Geometry: final body of the model. Coordinates: model frame, mm. Give positions to 0.01 mm unless a question says otherwise; leave off trailing zeros. Loops run counter-clockwise (first coordinate to the right, second up) from the corner with the lowest first, then second, coordinate; pieces in that order, holes last. Notation, with made-up numbers: (66.5, 71.25) -> (112.5, 71.25) arc R24 ccw to (112.5, 86.25) -> close; hole circle Ø7 at (70.5, -32). An arc over 180 degrees is marked (long way). One line per question, with ' | ' between items. Start each with the question number.
Item 1: Pin query (flat end, axial travel): P1, Ø0.9, axis at x = 2, z = -17, coming from the +Y side; P2, Ø0.9, axis at x = 1, y = 61, coming from the -Z side. Return the tip coordinate at first contact, or that it passes through.
Item 2: Section A-A on z = -3. Give the number of separate pieces and of enclosed holes in the cut face, then the cut area to 4 significant figures.
Item 3: Material intervals for line 1 along Z through (x, y) = (1.45, -81); line 2 along Z through (x, y) = (2.85, -53), sorted ascending. Write a range as [from, to].
Item 4: Section C-C on y = -57.5. Return loops of the section in (x, z).
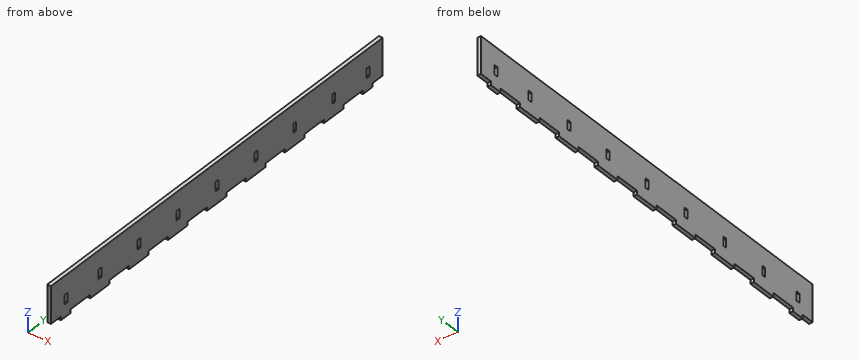
from build123d import *

# Parameters (mm, degrees)
F0_W      = 280
F0_H      = 30
F1_DEPTH  = 3
F2_W      = 20
F2_H      = 3
F3_DEPTH  = 3
F4_W      = 3
F4_H      = 7.5
F5_DEPTH  = 25
F6_W      = 30.25
F6_H      = 30
F7_DEPTH  = 3
F8_W      = 10
F8_H      = 3
F9_DEPTH  = 3
F10_W     = 3
F10_H     = 7.5
F11_DEPTH = 25


with BuildPart() as f1:
    # F0 (on Right) → F1 (new body)
    with BuildSketch(Plane.YZ):
        Rectangle(F0_W, F0_H)
    extrude(amount=F1_DEPTH)

    # F2 (on face) → F3 (join, through all)
    with BuildSketch(Plane.YZ.offset(3)):
        with Locations((120, -16.5)):
            Rectangle(F2_W, F2_H)
        with Locations((80, -16.5)):
            Rectangle(F2_W, F2_H)
        with Locations((40, -16.5)):
            Rectangle(F2_W, F2_H)
        with Locations((0, -16.5)):
            Rectangle(F2_W, F2_H)
        with Locations((-40, -16.5)):
            Rectangle(F2_W, F2_H)
        with Locations((-80, -16.5)):
            Rectangle(F2_W, F2_H)
        with Locations((-120, -16.5)):
            Rectangle(F2_W, F2_H)
    extrude(amount=-F3_DEPTH)

    # F4 (on face) → F5 (cut)
    with BuildSketch(Plane.YZ.offset(3)):
        with Locations((120, -3.75)):
            Rectangle(F4_W, F4_H)
        with Locations((80, -3.75)):
            Rectangle(F4_W, F4_H)
        with Locations((40, -3.75)):
            Rectangle(F4_W, F4_H)
        with Locations((0, -3.75)):
            Rectangle(F4_W, F4_H)
        with Locations((-40, -3.75)):
            Rectangle(F4_W, F4_H)
        with Locations((-80, -3.75)):
            Rectangle(F4_W, F4_H)
        with Locations((-120, -3.75)):
            Rectangle(F4_W, F4_H)
    extrude(amount=-F5_DEPTH, mode=Mode.SUBTRACT)

    # F6 (on face) → F7 (join)
    with BuildSketch(Plane.YZ.offset(3)):
        with Locations((-155.125, 0)):
            Rectangle(F6_W, F6_H)
        with Locations((155.125, 0)):
            Rectangle(F6_W, F6_H)
    extrude(amount=-F7_DEPTH)

    # F8 (on face) → F9 (join)
    with BuildSketch(Plane(origin=(0, 0, 0), x_dir=(0, -1, 0), z_dir=(-1, 0, 0))):
        with Locations((-155, -16.5)):
            Rectangle(F8_W, F8_H)
        with Locations((155, -16.5)):
            Rectangle(F8_W, F8_H)
    extrude(amount=-F9_DEPTH)

    # F10 (on face) → F11 (cut)
    with BuildSketch(Plane(origin=(0, 0, 0), x_dir=(0, -1, 0), z_dir=(-1, 0, 0))):
        with Locations((-155, -3.75)):
            Rectangle(F10_W, F10_H)
        with Locations((155, -3.75)):
            Rectangle(F10_W, F10_H)
    extrude(amount=-F11_DEPTH, mode=Mode.SUBTRACT)


solid = f1.part
Result sheet:
1) P1: stops at y = 160 | P2: stops at z = -15
2) separate pieces: 10 | enclosed holes: 0 | area: 940.5 mm²
3) line 1: z = [-18, -7.5], [0, 15] | line 2: z = [-15, 15]
4) outline: (0, -15) -> (3, -15) -> (3, 15) -> (0, 15) -> close
